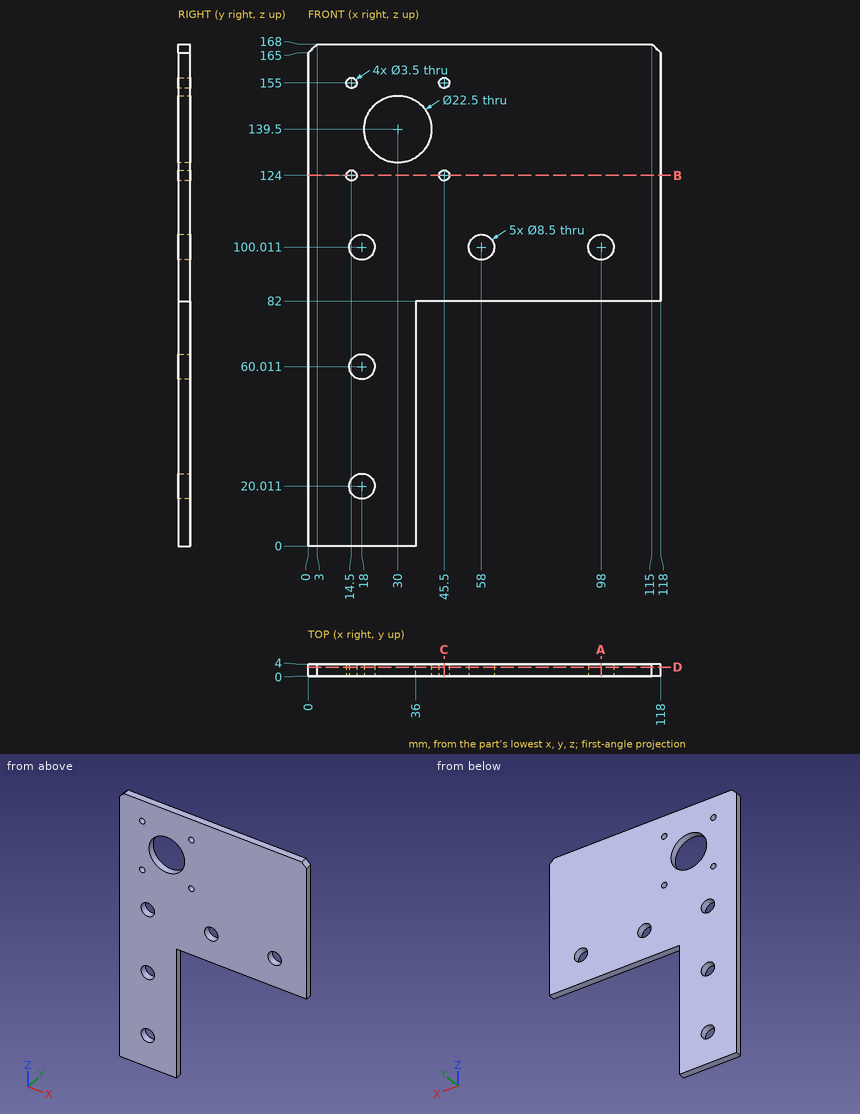
Study the drawing (mm; zero at the part's minimum x, y, z) and answer. Give positions to 0.01 mm unless a question says otherwise; leave off trailing zeros. Order: outer loops, then holes, each group sorted by start corner. A loop starts at its lowest first (then second) coordinate and runs counter-clockwise, first axis right, second up.
1. Straight lines are drawn through the part: L1, parallel to X at y = 3.15, z = 124; L2, parallel to X at y = 0.8, z = 72.5; L3, parallel to Z at x = 78.5, y = 2.35. For each, find the intervals that lie inside material, in ascending order.
Result sheet:
L1: x = 0 to 12.75, 16.25 to 43.75, 47.25 to 118
L2: x = 0 to 36
L3: z = 82 to 168
2. Section C-C, the plane x = 45.5 is taken. Determine the outline of the cut face in (y, z), and give its area (3 significant figures).
Result sheet:
outline: (0, 82) - (4, 82) - (4, 122.25) - (0, 122.25) - close; (0, 125.75) - (4, 125.75) - (4, 153.25) - (0, 153.25) - close; (0, 156.75) - (4, 156.75) - (4, 168) - (0, 168) - close
area: 316 mm2
3. Each of these flat-tipped pins is pushed along its axis until it touches: P1, Ø2, axis at y = 2.5, z = 29.5, coming from the +X side; P2, Ø1, axis at x = 58, y = 0.5, coming from the -Z side. Where does it stop, or does it pass through?
Result sheet:
P1: stops at x = 36
P2: stops at z = 82
4. Section B-B, the plane z = 124 is taken. Determine the outline of the cut face in (x, y).
Result sheet:
outline: (0, 0) - (12.75, 0) - (12.75, 4) - (0, 4) - close; (16.25, 0) - (43.75, 0) - (43.75, 4) - (16.25, 4) - close; (47.25, 0) - (118, 0) - (118, 4) - (47.25, 4) - close
5. Section D-D, the plane y = 2.95 is taken. Give the number of separate pieces and of enclosed holes in the cut face, and give its area (3 significant figures).
Result sheet:
separate pieces: 1
enclosed holes: 10
area: 12,400 mm2
6. Section A-A, the plane x = 98 is taken. Determine the outline of the cut face in (y, z), and give its area (3 significant figures).
Result sheet:
outline: (0, 82) - (4, 82) - (4, 95.76) - (0, 95.76) - close; (0, 104.26) - (4, 104.26) - (4, 168) - (0, 168) - close
area: 310 mm2
